```python
from build123d import *

# Parameters (mm, degrees)
SALIENTE_EXTRUIR1_DEPTH = 104
SALIENTE_EXTRUIR2_DEPTH = 1


with BuildPart() as part:
    # Croquis1 → Saliente-Extruir1 (new body)
    with BuildSketch(Plane.XY):
        Polygon((-55, 0), (-56.301708279, 0), (-32.968374946, 28), (32.968374946, 28), (56.301708279, 0), (55, 0), (32.5, 27), (-32.5, 27), align=None)
    extrude(amount=SALIENTE_EXTRUIR1_DEPTH)

    # Croquis4 → Saliente-Extruir2 (add)
    with BuildSketch(Plane.XY.offset(104)):
        Polygon((-56.301708279, 0), (56.301708279, 0), (32.968374946, 28), (-32.968374946, 28), align=None)
    extrude(amount=SALIENTE_EXTRUIR2_DEPTH)


solid = part.part
```
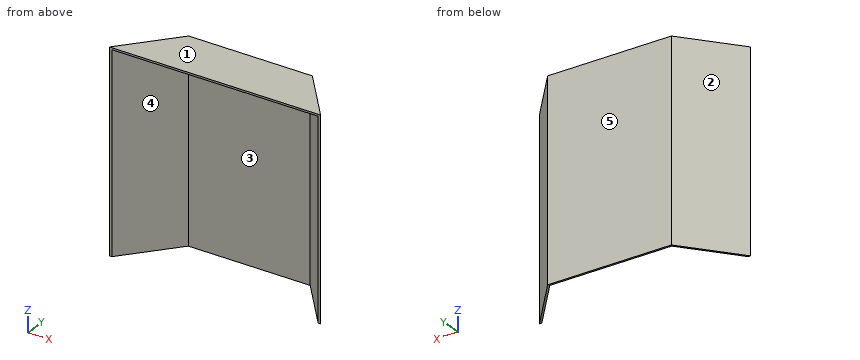
Geometry check sheet. Reference: the model listing, model coordinates, mm. Face numbers are marked on the shaded views. A direction names the side the tool comes from. Coordinates: 2 decimals unless noted, no trailing zeros. Order: outer loops, then holes, each group sorted by start corner. A loop starts at its lowest first (then second) coordinate and runs counter-clockwise, first axis right, second up. Notation, with made-up numbers: (12.25, -13.5) - (42.25, -13.5) arc R8 ccw to (42.25, -9.5) - close; hole circle Ø3 at (57, 4). An arc over 180 degrees is marked (long way). Answer as a JSON object with one key per item and string values. Group by question number.
Item 1: Draft check along X on the marked faces 1, 2 and 3. Enter one of: +X half, -X half, draft (parallel to the pull), parting line (faces both ways), or undercut.
Item 2: Tool access check on the marked faces 4 and 5. Record the directions out of +Z, -Z, +X, -X, +Y, -Y that give a thin tool (end or side, any length) a straight path to the whole face; none if there is none.
Item 3: Sectioned sample at B-B, the plane z = 87. Record the cut outline in (x, y), and give its area (3 significant figures).
Item 4: Sectioned sample at D-D, the plane x = -35. Record the cut outline in (y, z), and give its area (3 significant figures).
Item 5: Depth check by flat-ended pin: pin 1 Ø1 at (x, y) = (-16, 15.5) entering from -Z; pin 2 Ø4 at (x, z) = (-6, 29.5) entering from -Y; pin 3 Ø4 at (x, z) = (39.5, 91.5) entering from +Y. Enter the tip coordinate at first touch or a pass-through.
Item 6: Scan lines: probe 1 along Z at (x, y) = (-4, 23); probe 2 along X at (y, z) = (4.5, 43.5); probe 3 along Y at (x, z) = (9, 47). Record each from-to range of solid material in increasing order.
Item 7: Sectioned sample at A-A, the plane y = 21. Record the cut outline in (x, z), and give its area (3 significant figures).
Item 8: Sectioned sample at C-C, the plane x = -1. Record the cut outline in (y, z), and give its area (3 significant figures).
Resolved:
{
 "1": {"face 1": "draft", "face 2": "-X half", "face 3": "undercut"},
 "2": {"face 4": "-Z, -Y", "face 5": "+Z, -Z, +X, -X, +Y"},
 "3": {"outline": "(-56.3, 0) - (-55, 0) - (-32.5, 27) - (32.5, 27) - (55, 0) - (56.3, 0) - (32.97, 28) - (-32.97, 28) - close", "area": "137 mm^2"},
 "4": {"outline": "(0, 104) - (24, 104) - (24, 0) - (25.56, 0) - (25.56, 105) - (0, 105) - close", "area": "188 mm^2"},
 "5": {"pin 1": "z = 104", "pin 2": "y = 27", "pin 3": "y = 22.56"},
 "6": {"probe 1": "104 to 105", "probe 2": "-52.55 to -51.25, 51.25 to 52.55", "probe 3": "27 to 28"},
 "7": {"outline": "(-38.8, 0) - (-37.5, 0) - (-37.5, 104) - (37.5, 104) - (37.5, 0) - (38.8, 0) - (38.8, 105) - (-38.8, 105) - close", "area": "348 mm^2"},
 "8": {"outline": "(0, 104) - (27, 104) - (27, 0) - (28, 0) - (28, 105) - (0, 105) - close", "area": "132 mm^2"}
}
